Input: part model. Units: mm. Frame: model coordinates. A direction names the side the tool comes from. Coordinates: 2 decimals unless noted, no trailing zeros. Order: outer loops, then holes, each group sorted by start corner. A loop starts at its lowest first (then second) coordinate and runs counter-clockwise, first axis right, second up. Notation, with made-up numbers: (70.25, 21) -> (111.25, 21) arc R24 ccw to (111.25, 37) -> close; hole circle Ø5 at (25, 13). An arc over 180 degrees is marked (long way). Write each question's results on one line, items separated by ' | '.
```python
from build123d import *

# Parameters (mm, degrees)
SKETCH_1_W          = 150
SKETCH_1_H          = 110
EXTRUDE_1_DEPTH     = 8
SKETCH_2_R          = 1.75
CUT_EXTRUDE_1_DEPTH = 187.182705964
CUT_EXTRUDE_2_DEPTH = 187.182705964
SKETCH_4_W          = 110
SKETCH_4_H          = 20
CUT_EXTRUDE_3_DEPTH = 187.182705964
SKETCH_5_W          = 110
SKETCH_5_H          = 76
CUT_EXTRUDE_4_DEPTH = 5
FILLET_1_R          = 2
FILLET_2_R          = 3


with BuildPart() as part:
    # 草图1 → 凸台-拉伸1 (new body)
    with BuildSketch(Plane(origin=(0, 0, 0), x_dir=(1, 0, 0), z_dir=(0, 1, 0))):
        with Locations((75, 55)):
            Rectangle(SKETCH_1_W, SKETCH_1_H)
    extrude(amount=EXTRUDE_1_DEPTH)

    # 草图2 → 切除-拉伸1 (cut, through all)
    with BuildSketch(Plane(origin=(0, 8, 0), x_dir=(1, 0, 0), z_dir=(0, 1, 0))):
        with Locations(Location((4.6, 106, 0), (0, 0, 270))):
            Circle(SKETCH_2_R)
        with Locations(Location((4.6, 4, 0), (0, 0, 270))):
            Circle(SKETCH_2_R)
        with Locations(Location((104, 106, 0), (0, 0, 270))):
            Circle(SKETCH_2_R)
        with Locations(Location((146.8, 17, 0), (0, 0, 270))):
            Circle(SKETCH_2_R)
    extrude(amount=-CUT_EXTRUDE_1_DEPTH, mode=Mode.SUBTRACT)

    # 草图3 → 切除-拉伸2 (cut, through all)
    with BuildSketch(Plane(origin=(0, 8, 0), x_dir=(1, 0, 0), z_dir=(0, 1, 0))):
        with BuildLine():
            Line((102.25, 107.75), (105.75, 107.75))
            ThreePointArc((105.75, 107.75), (107.5, 106), (105.75, 104.25))
            Line((105.75, 104.25), (102.25, 104.25))
            ThreePointArc((102.25, 104.25), (100.5, 106), (102.25, 107.75))
        make_face()
        with BuildLine():
            Line((145.05, 15.25), (145.05, 18.75))
            ThreePointArc((145.05, 18.75), (146.8, 20.5), (148.55, 18.75))
            Line((148.55, 18.75), (148.55, 15.25))
            ThreePointArc((148.55, 15.25), (146.8, 13.5), (145.05, 15.25))
        make_face()
    extrude(amount=-CUT_EXTRUDE_2_DEPTH, mode=Mode.SUBTRACT)

    # 草图4 → 切除-拉伸3 (cut, through all)
    with BuildSketch(Plane(origin=(0, 8, 0), x_dir=(1, 0, 0), z_dir=(0, 1, 0))):
        with Locations((87, 33)):
            Rectangle(SKETCH_4_W, SKETCH_4_H)
    extrude(amount=-CUT_EXTRUDE_3_DEPTH, mode=Mode.SUBTRACT)

    # 草图5 → 切除-拉伸4 (cut)
    with BuildSketch(Plane(origin=(0, 8, 0), x_dir=(1, 0, 0), z_dir=(0, 1, 0))):
        with Locations((87, 61)):
            Rectangle(SKETCH_5_W, SKETCH_5_H)
    extrude(amount=-CUT_EXTRUDE_4_DEPTH, mode=Mode.SUBTRACT)

    # 圆角1
    fillet_1_edges = [part.edges().sort_by_distance(p)[0] for p in [
        (32, 4, -23),
        (32, 1.5, -43),
        (142, 1.5, -43),
        (142, 4, -23),
    ]]
    fillet(fillet_1_edges, radius=FILLET_1_R)

    # 圆角2
    fillet_2_edges = [part.edges().sort_by_distance(p)[0] for p in [
        (0, 4, -110),
        (150, 4, -110),
        (150, 4, 0),
        (0, 4, 0),
    ]]
    fillet(fillet_2_edges, radius=FILLET_2_R)


solid = part.part
```
(1) Reachability of faces 4 (the face through (86, 4, -23)), 5 (the face through (0.9, 4.06, -0.86)), 6 (the face through (86, 3, -70)) from +Z, -Z, +X, -X, +Y, -Y: full face, straight path, thin tool, end or side. Return the list, or none.
Return value:
face 4: +Y, -Y | face 5: +Z, -X, +Y, -Y | face 6: +Y
(2) Cut plane C-C, the plane y = 1.75. Return loops of the section in (x, z), plus the area to 3 significant figures.
Return value:
outline: (0, -107) arc R3 ccw to (3, -110) -> (147, -110) arc R3 ccw to (150, -107) -> (150, -3) arc R3 ccw to (147, 0) -> (3, 0) arc R3 ccw to (0, -3) -> close; hole circle Ø3.5 at (4.6, -106); hole circle Ø3.5 at (4.6, -4); hole (32, -41) arc R2 ccw to (34, -43) -> (140, -43) arc R2 ccw to (142, -41) -> (142, -25) arc R2 ccw to (140, -23) -> (34, -23) arc R2 ccw to (32, -25) -> close; hole (102.25, -107.75) -> (105.75, -107.75) arc R1.75 ccw to (105.75, -104.25) -> (102.25, -104.25) arc R1.75 ccw to start; hole (145.05, -18.75) arc R1.75 ccw to (148.55, -18.75) -> (148.55, -15.25) arc R1.75 ccw to (145.05, -15.25) -> close | area: 14,200 mm2
(3) Line query: line 1 along Z through (x, y) = (103, 1.5); line 2 along Z through (x, y) = (103, 7.25); line 3 along X through (y, z) = (6.5, -106). Output: solid intervals per line, ascending. Write a range as from..to.
Return value:
line 1: -110..-107.75, -104.25..-43, -23..0 | line 2: -110..-107.75, -104.25..-99, -23..0 | line 3: 0..2.85, 6.35..100.5, 107.5..150
(4) Cut plane A-A, the plane x = 94.5. Return loops of the section in (y, z).
Return value:
outline: (0, -110) -> (8, -110) -> (8, -99) -> (3, -99) -> (3, -43) -> (0, -43) -> close; (0, -23) -> (8, -23) -> (8, 0) -> (0, 0) -> close
(5) Mould query, pull axis Z, two halves, no side actions, for faces 1 (the face through (5.78, 4.06, -5.29)), 2 (the face through (0, 4, -54)), 3 (the face through (74, 4, 0)). Classes: +Z half, -Z half, draft (parallel to the pull), parting line (faces both ways), or undercut.
Return value:
face 1: undercut | face 2: draft | face 3: +Z half
(6) Pin query (flat end, axial travel): P1, Ø5.5, axis at x = 4.6, z = -106, coming from the -Y side; P2, Ø8, axis at x = 115.5, z = -57.5, coming from the +Y side. Return the tip coordinate at first contact, or that it passes through.
Return value:
P1: y = 0 | P2: y = 3
(7) Cut plane B-B, the plane z = -30. Return loops of the section in (x, y).
Return value:
outline: (0, 0) -> (32, 0) -> (32, 8) -> (0, 8) -> close; (142, 0) -> (150, 0) -> (150, 8) -> (142, 8) -> close
